from build123d import *

# Parameters (mm, degrees)
F0_R     = 25.25
F1_DEPTH = 18


with BuildPart() as f1:
    # F0 (on Top) → F1 (new body)
    with BuildSketch(Plane.XY):
        with BuildLine():
            Line((-9.5, 55), (-9.5, 74.3959))
            ThreePointArc((-9.5, 74.3959), (-44.083894, 60.676275), (-67.819044, 32.024634))
            Line((-67.819044, 32.024634), (-49.372447, 26.030972))
            Line((-49.372447, 26.030972), (-55.24377, 7.960898))
            Line((-55.24377, 7.960898), (-73.690367, 13.954561))
            ThreePointArc((-73.690367, 13.954561), (-71.329239, -23.176275), (-51.414475, -54.603588))
            Line((-51.414475, -54.603588), (-40.01385, -38.911975))
            Line((-40.01385, -38.911975), (-24.642527, -50.079895))
            Line((-24.642527, -50.079895), (-36.043152, -65.771508))
            ThreePointArc((-36.043152, -65.771508), (0, -75), (36.043152, -65.771508))
            Line((36.043152, -65.771508), (24.642527, -50.079895))
            Line((24.642527, -50.079895), (40.01385, -38.911975))
            Line((40.01385, -38.911975), (51.414475, -54.603588))
            ThreePointArc((51.414475, -54.603588), (71.329239, -23.176275), (73.690367, 13.954561))
            Line((73.690367, 13.954561), (55.24377, 7.960898))
            Line((55.24377, 7.960898), (49.372447, 26.030972))
            Line((49.372447, 26.030972), (67.819044, 32.024634))
            ThreePointArc((67.819044, 32.024634), (44.083894, 60.676275), (9.5, 74.3959))
            Line((9.5, 74.3959), (9.5, 55))
            Line((9.5, 55), (-9.5, 55))
        make_face()
        with Locations((-0.347831, 0.255336)):
            Circle(F0_R, mode=Mode.SUBTRACT)
    extrude(amount=F1_DEPTH)


solid = f1.part
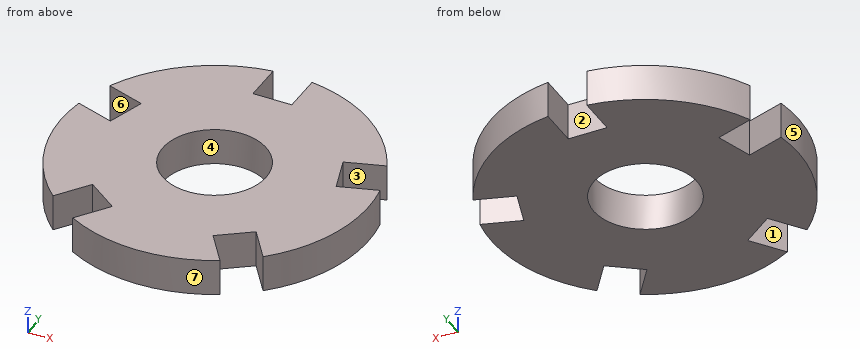
Source: CAD feature listing. Evaluate the final solid. Frame: model axes, mm. Face numbers are marked on the shaded views. A direction names the side the tool comes from. Round coordinates to 2 decimals unless told otherwise and drop trailing zeros. Loops run counter-clockwise (first coordinate to the right, second up) from the corner with the lowest first, then second, coordinate; pieces in that order, holes last. Notation, with made-up numbers: (-13.75, 8) - (40.25, 8) arc R20 cw to (40.25, 13) - close; hole circle Ø6 at (22.25, 75.5). An arc over 180 degrees is marked (long way). Write item = value, one per line. Start each with the question number.
(1) Ray query, line 1 along X through (y, z) = (-0.5, 14.25); line 2 along Y through (x, z) = (-2.5, 16.5); line 3 along X through (y, z) = (-12.5, 6.75). Return the intervals inside material, ascending. Write a range as from..to.
(2) Section query D-D, the plane y = -45. Output: boundary loops of the cut face in (x, z).
(3) Set-up query: the marked faces 1, 2 and 3. Return all of +Z, -Z, +X, -X, +Y, -Y with unobstructed straight access to the full face (end or side cutting, diameter ignored); none if empty.
(4) Pull-direction query (Y, two-part tool) for the marked faces 4, 5, 6 and 7; classes: +Y half, -Y half, draft (parallel to the pull), parting line (faces both ways), or undercut.
(5) Pin query (flat end, axial travel): pin 1 (8 mm diameter, centred on x = 50.5, z = 8, fed in from -Y); pin 2 (2 mm diameter, centred on x = -57, z = 11, fed in from -Y); pin 3 (5 mm diameter, centred on x = -0.5, z = 11.5, fed in from +Y); pin 4 (6 mm diameter, centred on x = 12.5, y = 41, fed in from -Z). Return the tip coordinate at first contact, or that it passes through.
(6) Section query B-B, the plane x = -22. Output: boundary loops of the cut face in (y, z).
(7) Section query C-C, the plane z = 12. Output: boundary loops of the cut face in (x, y).
(8) Section query A-A, the plane y = 22.5. Output: boundary loops of the cut face in (x, z).
Conclusion:
q1.line_1 = -75..-25.59, 24.89..75
q1.line_2 = -74.96..-24.9, 25.41..55
q1.line_3 = -73.95..-22.14, 21.44..73.95
q2.outline = (-60, 0) - (-44.44, 0) - (-44.44, 18) - (-60, 18) - close; (-31.63, 0) - (31.63, 0) - (31.63, 18) - (-31.63, 18) - close; (44.44, 0) - (60, 0) - (60, 18) - (44.44, 18) - close
q3.face_1 = +Z, -Z
q3.face_2 = +Z, -Z, +Y
q3.face_3 = +Z, -Z, +X
q4.face_4 = undercut
q4.face_5 = parting line
q4.face_6 = undercut
q4.face_7 = -Y half
q5.pin_1 = -54.6
q5.pin_2 = -49.89
q5.pin_3 = 55
q5.pin_4 = 0
q6.outline = (-71.7, 0) - (-12.73, 0) - (-12.73, 18) - (-71.7, 18) - close; (13.25, 0) - (71.7, 0) - (71.7, 18) - (13.25, 18) - close
q7.outline = (-73.69, 13.95) arc R75 ccw to (-51.41, -54.6) - (-40.01, -38.91) - (-24.64, -50.08) - (-36.04, -65.77) arc R75 ccw to (36.04, -65.77) - (24.64, -50.08) - (40.01, -38.91) - (51.41, -54.6) arc R75 ccw to (73.69, 13.95) - (55.24, 7.96) - (49.37, 26.03) - (67.82, 32.02) arc R75 ccw to (9.5, 74.4) - (9.5, 55) - (-9.5, 55) - (-9.5, 74.4) arc R75 ccw to (-67.82, 32.02) - (-49.37, 26.03) - (-55.24, 7.96) - close; hole circle Ø50.5 at (-0.35, 0.26)
q8.outline = (-50.52, 0) - (-12.3, 0) - (-12.3, 18) - (-50.52, 18) - close; (11.6, 0) - (50.52, 0) - (50.52, 18) - (11.6, 18) - close
